```python
from build123d import *

# Parameters (mm, degrees)
SKETCH1_R           = 2.25
BOSS_EXTRUDE1_DEPTH = 12.7
SKETCH3_R           = 4.35
CUT_EXTRUDE1_DEPTH  = 43.816935902
CUT_EXTRUDE2_START  = 12.7
SKETCH1_3_R         = 2.25
CUT_EXTRUDE2_DEPTH  = 8
CUT_EXTRUDE4_START  = -12.7
SKETCH1_5_R         = 2.25
CUT_EXTRUDE4_DEPTH  = 8
CUT_EXTRUDE3_START  = -9
SKETCH3_3_R         = 4.35
CUT_EXTRUDE3_DEPTH  = 34.816936066


with BuildPart() as part:
    # Sketch1 → Boss-Extrude1 (new, symmetric)
    with BuildSketch(Plane.XY):
        with BuildLine():
            ThreePointArc((-26.566778815, 17.838336901), (0, 32), (26.566778815, 17.838336901))
            Line((26.566778815, 17.838336901), (13.258035703, 10.154530482))
            ThreePointArc((13.258035703, 10.154530482), (0, 16.7), (-13.258035703, 10.154530482))
            Line((-13.258035703, 10.154530482), (-26.566778815, 17.838336901))
        make_face()
        with Locations((17.67766953, 17.67766953)):
            Circle(SKETCH1_R, mode=Mode.SUBTRACT)
        with Locations((-17.67766953, 17.67766953)):
            Circle(SKETCH1_R, mode=Mode.SUBTRACT)
        with Locations((-17.67766953, 17.67766953)):
            Circle(SKETCH1_R)
        with Locations((17.67766953, 17.67766953)):
            Circle(SKETCH1_R)
    extrude(amount=BOSS_EXTRUDE1_DEPTH, both=True)

    # Sketch3 → Cut-Extrude1 (cut, symmetric)
    with BuildSketch(Plane(origin=(-1.082531755, 1.875, 0), x_dir=(0.8660254037844398, 0.4999999999999983, 0), z_dir=(0.4999999999999983, -0.8660254037844398, 0))):
        with Locations((22.059060964, 0)):
            Circle(SKETCH3_R)
    cut_extrude1 = extrude(amount=CUT_EXTRUDE1_DEPTH, both=True, mode=Mode.SUBTRACT)

    # Sketch1<3> → Cut-Extrude2 (cut)
    with BuildSketch(Plane.XY.offset(CUT_EXTRUDE2_START)):
        with Locations((17.67766953, 17.67766953)):
            Circle(SKETCH1_3_R)
    cut_extrude2 = extrude(amount=-CUT_EXTRUDE2_DEPTH, mode=Mode.SUBTRACT)

    # Sketch1<5> → Cut-Extrude4 (cut)
    with BuildSketch(Plane.XY.offset(CUT_EXTRUDE4_START)):
        with Locations((17.67766953, 17.67766953)):
            Circle(SKETCH1_5_R)
    cut_extrude4 = extrude(amount=CUT_EXTRUDE4_DEPTH, mode=Mode.SUBTRACT)

    # Sketch3<3> → Cut-Extrude3 (cut, through all)
    with BuildSketch(Plane(origin=(-1.082531755, 1.875, 0), x_dir=(0.8660254037844398, 0.4999999999999983, 0), z_dir=(0.4999999999999983, -0.8660254037844398, 0)).offset(CUT_EXTRUDE3_START)):
        Polygon((18.23411543, -6.625), (25.884006497, -6.625), (29.70895203, 0), (25.884006497, 6.625), (18.23411543, 6.625), (14.409169897, 0), align=None)
        with Locations((22.059060964, 0)):
            Circle(SKETCH3_3_R, mode=Mode.SUBTRACT)
    cut_extrude3 = extrude(amount=-CUT_EXTRUDE3_DEPTH, mode=Mode.SUBTRACT)

    # Mirror1: Cut-Extrude1, Cut-Extrude2, Cut-Extrude4, Cut-Extrude3 across plane
    add(cut_extrude1.mirror(Plane(origin=(0, 0, 0), x_dir=(0, 0, 1), z_dir=(1, 0, 0))), mode=Mode.SUBTRACT)
    add(cut_extrude2.mirror(Plane(origin=(0, 0, 0), x_dir=(0, 0, 1), z_dir=(1, 0, 0))), mode=Mode.SUBTRACT)
    add(cut_extrude4.mirror(Plane(origin=(0, 0, 0), x_dir=(0, 0, 1), z_dir=(1, 0, 0))), mode=Mode.SUBTRACT)
    add(cut_extrude3.mirror(Plane(origin=(0, 0, 0), x_dir=(0, 0, 1), z_dir=(1, 0, 0))), mode=Mode.SUBTRACT)


solid = part.part
```
Verification items for the finished model (mm, model axes). A direction names the side the tool comes from. Round coordinates to 2 decimals unless told otherwise and drop trailing zeros. Order: outer loops, then holes, each group sorted by start corner. A loop starts at its lowest first (then second) coordinate and runs counter-clockwise, first axis right, second up. Notation, with made-up numbers: (-23, 27) -> (-10, 27) arc R12 ccw to (-10, 45) -> close; hole circle Ø6 at (86, 47). An arc over 180 degrees is marked (long way). Put each result on its own line as item: value. Start each with the question number.
(1) Tool access check on faces 4 (the face through (-13.428, 20.645, 4.509)), 5 (the face through (-18.716, 15.682, 8.756)), 6 (the face through (-18, 18, -4.7)), 7 (the face through (-4.45, 24.882, -3.266)). Record the directions out of +Z, -Z, +X, -X, +Y, -Y that give a thin tool (end or side, any length) a straight path to the whole face; none if there is none.
(2) Draft check along Z on faces 1 (the face through (18, 18, 4.7)), 2 (the face through (18, 18, -4.7)), 3 (the face through (-19.396, 18.822, 1.307)). Enter one of: +Z half, -Z half, draft (parallel to the pull), parting line (faces both ways), or undercut.
(3) Material ranges on line 1 along X through (y, z) = (24, 2.5); line 2 along X through (y, z) = (22.5, 1.5); line 3 along Z through (x, y) = (10, 24.5) (3 decimals), recorded low to high.
(4) Section check B-B (z = 6). Enter the section's corners in (x, y), then the cut area to 3 significant figures.
(5) Depth check by flat-ended pin: pin 1 Ø6 at (x, z) = (1, -1.5) entering from -Y; pin 2 Ø2 at (y, z) = (22.5, 2.5) entering from +X; pin 3 Ø3.5 at (x, y) = (18, 17.5) entering from -Z. Enter the tip coordinate at first touch or a pass-through.
(6) Section check D-D (z = -1.25). Enter the section's corners in (x, y), then the cut area to 3 significant figures.
(7) Section check A-A (y = 30.5). Enter the section's corners in (x, z) (3 decimals).
(8) Section check C-C (x = 4). Enter the section's corners in (y, z) (3 decimals).
Completed:
1. face 4: none
1. face 5: +Z
1. face 6: -Z
1. face 7: +Y
2. face 1: +Z half
2. face 2: -Z half
2. face 3: undercut
3. line 1: x = -21.17 to -18.78, -4.45 to 4.45, 18.78 to 21.17
3. line 2: x = -22.75 to -17.2, -4.65 to 4.65, 17.2 to 22.75
3. line 3: z = -12.7 to -6.625, 6.625 to 12.7
4. outline: (-26.57, 17.84) -> (-13.26, 10.15) arc R16.7 cw to (13.26, 10.15) -> (26.57, 17.84) arc R32 ccw to (13.57, 28.98) -> (17.15, 22.79) -> (9.9, 18.61) -> (2.21, 31.92) arc R32 ccw to (-2.21, 31.92) -> (-9.9, 18.61) -> (-17.15, 22.79) -> (-13.57, 28.98) arc R32 ccw to start; hole circle Ø4.5 at (-17.68, 17.68); hole circle Ø4.5 at (17.68, 17.68)
4. area: 485 mm2
5. pin 1: stops at y = 16.21
5. pin 2: stops at x = 23.7
5. pin 3: stops at z = -4.7
6. outline: (-26.57, 17.84) -> (-21.63, 14.99) -> (-17.13, 22.78) -> (-19.52, 24.16) -> (-18.33, 26.23) arc R32 ccw to start; (-14.41, 10.82) -> (-13.26, 10.15) arc R16.7 cw to (13.26, 10.15) -> (14.41, 10.82) -> (9.91, 18.62) -> (7.52, 17.23) -> (0, 30.26) -> (-7.52, 17.23) -> (-9.91, 18.62) -> close; (17.13, 22.78) -> (21.63, 14.99) -> (26.57, 17.84) arc R32 ccw to (18.33, 26.23) -> (19.52, 24.16) -> close
6. area: 253 mm2
7. outline: (-9.682, -12.7) -> (9.682, -12.7) -> (9.682, -6.625) -> (3.446, -6.625) -> (0, -1.456) -> (-3.446, -6.625) -> (-9.682, -6.625) -> close; (-9.682, 6.625) -> (-3.446, 6.625) -> (0, 1.456) -> (3.446, 6.625) -> (9.682, 6.625) -> (9.682, 12.7) -> (-9.682, 12.7) -> close
8. outline: (16.214, -12.7) -> (31.749, -12.7) -> (31.749, -6.625) -> (29.54, -6.625) -> (21.89, 0) -> (29.54, 6.625) -> (31.749, 6.625) -> (31.749, 12.7) -> (16.214, 12.7) -> close
